The listing builds one solid part. Answer for the finished solid, in the listing's coordinates (mm). Face numbers are marked on the shaded views. A direction names the side the tool comes from. Give positions to 0.01 mm unless a question says otherwise; leave off trailing zeros. Loops run counter-clockwise (first coordinate to the right, second up) from the corner with the lowest first, then second, coordinate; pieces in that order, holes last. Notation, with made-up numbers: (88.25, 45) -> (125.25, 45) arc R12 ccw to (125.25, 62) -> close; hole circle Ø4 at (34.5, 33.5). An arc over 180 degrees is marked (long way). One line per question, with ' | ' between items. Start each with the question number.
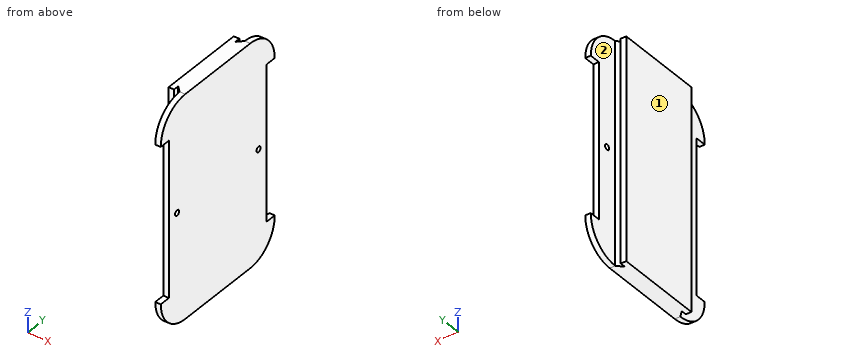
Autodesk Inventor part; units mm, degrees
ref_plane "YZ Plane" through (0, 0, 0) normal (1, 0, 0) x (0, 1, 0)
ref_plane "XZ Plane" through (0, 0, 0) normal (0, 1, 0) x (-1, 0, 0)
ref_plane "XY Plane" through (0, 0, 0) normal (0, 0, 1) x (1, 0, 0)
sketch "Sketch1" plane through (0, 0, 0) normal (1, 0, 0) x (0, 1, 0)
  line L0 (-76.2, 88.9) -> (-76.2, 88.9)
  line L1 (-50.8, 127) -> (50.8, 127)
  line L2 (50.8, -127) -> (-50.8, -127)
  line L3 (-76.2, -88.9) -> (-76.2, 88.9)
  arc A0 (88.9, 88.9) -> (50.8, 127) centre (50.8, 88.9) ccw
  line L4 (76.2, 88.9) -> (88.9, 88.9)
  arc A1 (-50.8, 127) -> (-88.9, 88.9) centre (-50.8, 88.9) ccw
  line L5 (-50.8, 88.9) -> (-88.9, 88.9)
  arc A2 (50.8, -127) -> (88.9, -88.9) centre (50.8, -88.9) ccw
  line L6 (76.2, -88.9) -> (88.9, -88.9)
  line L7 (76.2, 88.9) -> (76.2, -88.9)
  arc A3 (-88.9, -88.9) -> (-50.8, -127) centre (-50.8, -88.9) ccw
  line L8 (-76.2, -88.9) -> (-88.9, -88.9)
  point P0 (0, 0)
  point P1 (-76.2, 117.2981)
  point P2 (-76.2, -117.2981)
  dimension "d62" = 254
  dimension "d64" = 76.2
  dimension "d65" = 127
  dimension "d66" = 76.2
  dimension "d72" = 76.2
  dimension "d73" = 25.4
  dimension "d74" = 76.2
  dimension "d76" = 25.4
  dimension "d77" = 76.2
  dimension "d78" = 25.4
extrude "Extrusion1" add sketch "Sketch1" along normal blind 6.35
sketch "Sketch3" plane through (6.35, 0, 0) normal (1, 0, 0) x (0, 0, -1)
  line L0 (88.9, 76.2) -> (-88.9, 76.2)
  line L1 (127, -50.8) -> (127, 50.8)
  line L2 (-88.9, -76.2) -> (88.9, -76.2)
  point P0 (0, 0)
  point P1 (0, -63.5)
  point P2 (0, 63.5)
  point P3 (0, 63.5)
  point P4 (127, 76.2)
  point P5 (127, -76.2)
  point P6 (-127, -76.2)
  dimension "d68" = 12.7
  dimension "d69" = 127
  dimension "d70" = 127
  dimension "d71" = 12.7
hole "Hole2" at (6.35, -63.5, 0) direction (-1, 0, 0) diameter 6.35 end through all
hole "Hole3" at (6.35, 63.5, 0) direction (-1, 0, 0) diameter 6.35 end through all
sketch "Sketch4" plane through (6.35, 0, 0) normal (1, 0, 0) x (0, 0, -1)
  line L0 (-127, 50.8) -> (-127, -50.8)
  line L1 (-127, 50.8) -> (127, 50.8)
  line L2 (127, 50.8) -> (127, -50.8)
  line L3 (127, -50.8) -> (-127, -50.8)
  line L4 (-127, -50.8) -> (-127, 50.8)
  point P0 (0, 0)
  point P1 (-88.9, 88.9)
  dimension "d79" = 101.6
  dimension "d80" = 38.1
extrude "Extrusion2" add sketch "Sketch4" against normal blind 19.05
sketch "Sketch6" plane through (6.35, -50.8, -127) normal (0, 0, -1) x (-1, 0, 0)
  line L0 (6.35, 0) -> (0, 0)
  line L1 (6.35, 0) -> (12.7, 6.35)
  line L2 (6.35, 0) -> (15.3303, 0) construction
  line L3 (12.7, 6.35) -> (12.7, 0)
  line L4 (12.7, 0) -> (6.35, 0)
  point P0 (6.35, 50.8)
  dimension "d84" = 45
  dimension "d85" = 6.35
extrude "Extrusion3" cut sketch "Sketch6" against normal up to next
sketch "Sketch7" plane through (6.35, -50.8, -127) normal (0, 0, -1) x (-1, 0, 0)
  line L0 (6.35, 101.6) -> (19.05, 101.6)
  line L1 (6.35, 101.6) -> (12.7, 101.6)
  line L2 (12.7, 101.6) -> (12.7, 95.25)
  line L3 (12.7, 95.25) -> (6.35, 101.6)
  point P0 (6.35, 50.8)
  dimension "d92" = 6.35
extrude "Extrusion4" cut sketch "Sketch7" against normal up to next
properties part number "Frame" material "ABS Plastic"
1. Each of these flat-tipped pins is pushed along its axis until it touches: pin 1 Ø5.5 at (y, z) = (-63.5, 0) entering from -X; pin 2 Ø7 at (x, y) = (1.5, -79.5) entering from -Z; pin 3 Ø3 at (x, z) = (-8, -29) entering from +Y; pin 4 Ø3 at (x, z) = (-9, 3) entering from -Y. Where does it stop, or does it pass through?
2. For the marked faces 1 and 2, determine the directions among +Z, -Z, +X, -X, +Y, -Y from which every point of the face is accessible in a straight line to the end or side of a thin tool.
3. The part is cut by section C-C (z = 109.5). Write down the section's boundary in (x, y), plus the area to 3 significant figures.
4. The part is cut by section A-A (z = 0). Write down the section's boundary in (x, y) (3 decimals), plus the area to 3 significant figures.
5. The part is cut by section B-B (y = 63.5). Write down the section's boundary in (x, z) (3 decimals), plus the area to 3 significant figures.
6. Straight lines are drawn through the part: L1, parallel to Y at x = 4.5, z = 0 (3 decimals); L2, parallel to Y at x = -9, z = -71; L3, parallel to X at y = 68.5, z = -89.5. For each, find the intervals that lie inside material, in ascending order.
Check sheet entries:
1) pin 1: passes through | pin 2: stops at z = -117.48 | pin 3: stops at y = 50.8 | pin 4: stops at y = -50.8
2) face 1: +Z, -Z, -X, +Y, -Y | face 2: +Z, -Z, -X, +Y
3) outline: (-12.7, -50.8) -> (-6.35, -50.8) -> (-6.35, -44.45) -> (0, -50.8) -> (0, -82.85) -> (6.35, -82.85) -> (6.35, 82.85) -> (0, 82.85) -> (0, 50.8) -> (-6.35, 44.45) -> (-6.35, 50.8) -> (-12.7, 50.8) -> close | area: 2,300 mm^2
4) outline: (-12.7, -50.8) -> (-6.35, -50.8) -> (-6.35, -44.45) -> (0, -50.8) -> (0, -60.325) -> (6.35, -60.325) -> (6.35, 60.325) -> (0, 60.325) -> (0, 50.8) -> (-6.35, 44.45) -> (-6.35, 50.8) -> (-12.7, 50.8) -> close; (0, -76.2) -> (6.35, -76.2) -> (6.35, -66.675) -> (0, -66.675) -> close; (0, 66.675) -> (6.35, 66.675) -> (6.35, 76.2) -> (0, 76.2) -> close | area: 2,140 mm^2
5) outline: (0, -124.821) -> (6.35, -124.821) -> (6.35, -3.175) -> (0, -3.175) -> close; (0, 3.175) -> (6.35, 3.175) -> (6.35, 124.821) -> (0, 124.821) -> close | area: 1,540 mm^2
6) L1: y = -76.2 to -66.675, -60.325 to 60.325, 66.675 to 76.2 | L2: y = -50.8 to 50.8 | L3: x = 0 to 6.35
